```python
from build123d import *

# Parameters (mm, degrees)
HOLE1_D                      = 40
HOLE1_CBORE_D                = 70
HOLE1_CBORE_DEPTH            = 15
SKETCH4_R                    = 68
SKETCH4_R_2                  = 62
CUT_EXTRUDE1_DEPTH           = 3
FILLET1_R                    = 21
FILLET2_R                    = 12
BOSS_EXTRUDE1_START          = -10
BOSS_EXTRUDE1_DEPTH          = 10
CIRPATTERN1_COUNT            = 5
M10_TAPPED_HOLE1_D           = 8.5
M10_TAPPED_HOLE1_DEPTH       = 21.946342369
M10_TAPPED_HOLE1_CSINK_D     = 10.05
M10_TAPPED_HOLE1_CSINK_ANGLE = 90
M10_TAPPED_HOLE1_TIP         = 2.553657631


with BuildPart() as part:
    # Sketch1 → Revolve1 (revolve)
    with BuildSketch(Plane.XY, mode=Mode.PRIVATE) as revolve1_sk:
        Polygon((0, 0), (0, 90), (-85, 90), (-85, 80), (-40, 80), (-40, 6), (-50, 6), (-50, 0), align=None)
    revolve(revolve1_sk.sketch.rotate(Axis((0, 0, 0), (0, 1, 0)), 270), axis=Axis((0, 0, 0), (0, 1, 0)))

    # Hole1 (through all)
    with Locations(Plane(origin=(0, 90, 0), x_dir=(1, 0, 0), z_dir=(0, 1, 0))):
        with Locations((0, 0)):
            CounterBoreHole(HOLE1_D / 2, HOLE1_CBORE_D / 2, HOLE1_CBORE_DEPTH)

    # Sketch4 → Cut-Extrude1 (cut)
    with BuildSketch(Plane(origin=(0, 90, 0), x_dir=(1, 0, 0), z_dir=(0, 1, 0))):
        with Locations(Location((0, 0, 0), (0, 0, 270))):
            Circle(SKETCH4_R)
        with Locations(Location((0, 0, 0), (0, 0, 270))):
            Circle(SKETCH4_R_2, mode=Mode.SUBTRACT)
    extrude(amount=-CUT_EXTRUDE1_DEPTH, mode=Mode.SUBTRACT)

    # Fillet1
    fillet1_edges = [part.edges().sort_by_distance(p)[0] for p in [
        (0, 80, 40),
    ]]
    fillet(fillet1_edges, radius=FILLET1_R)

    # Fillet2
    # the kernel refuses this fillet: 12 mm, written as the material it adds along each edge
    with BuildSketch(Plane(origin=(0, 6, 0), x_dir=(0, 0, -1), z_dir=(1, 0, 0))) as fillet2_piece_1:
        with BuildLine():
            CenterArc((52, 11.832159566), FILLET2_R, 180, 80.405931773)
            Line((50, 0), (49.96, -0.236643191))
            ThreePointArc((49.96, -0.236643191), (45, -0.24), (40, -0.24))
            Line((40, -0.24), (39.76, 0))
            Line((39.76, 0), (39.76, 11.832159566))
            Line((39.76, 11.832159566), (40, 11.832159566))
        make_face()
    revolve(axis=Axis((0, 6, 0), (0, 1, 0)))

    # Sketch5 → Boss-Extrude1 (add)
    with BuildSketch(Plane(origin=(0, 90, 0), x_dir=(1, 0, 0), z_dir=(0, 1, 0)).offset(BOSS_EXTRUDE1_START)):
        with BuildLine():
            ThreePointArc((12.466163113, 84.080882353), (0, 97.5), (-12.466163113, 84.080882353))
            ThreePointArc((-12.466163113, 84.080882353), (0, 85), (12.466163113, 84.080882353))
        make_face()
    boss_extrude1 = extrude(amount=BOSS_EXTRUDE1_DEPTH)

    # CirPattern1: Boss-Extrude1 ×5 about axis
    cirpattern1_axis = Axis((0, 0, 0), (0, 1, 0))
    for i in range(1, CIRPATTERN1_COUNT):
        add(boss_extrude1.rotate(cirpattern1_axis, i * 360 / CIRPATTERN1_COUNT))

    # M10 Tapped Hole1
    with Locations(Plane(origin=(0, 90, 0), x_dir=(1, 0, 0), z_dir=(0, 1, 0))):
        with Locations((49.961746445, -68.766444522), (-49.961746445, -68.766444522), (80.839803885, 26.266444522), (0, 85), (-80.839803885, 26.266444522)):
            CounterSinkHole(M10_TAPPED_HOLE1_D / 2, M10_TAPPED_HOLE1_CSINK_D / 2, depth=M10_TAPPED_HOLE1_DEPTH, counter_sink_angle=M10_TAPPED_HOLE1_CSINK_ANGLE)
            with Locations((0, 0, -(M10_TAPPED_HOLE1_DEPTH + M10_TAPPED_HOLE1_TIP / 2))):  # 118° drill point
                Cone(0, M10_TAPPED_HOLE1_D / 2, M10_TAPPED_HOLE1_TIP, mode=Mode.SUBTRACT)


solid = part.part
```
CAD build for the part. Positions are in the model's coordinates, mm. A direction names the side the tool comes from. Give positions to 0.01 mm unless a question says otherwise; leave off trailing zeros. Loops run counter-clockwise (first coordinate to the right, second up) from the corner with the lowest first, then second, coordinate; pieces in that order, holes last. Notation, with made-up numbers: M -33,-17.75 L -18,-17.75 A28 cw -18,16.25 Z; hole C 9.25,25.25 d5. An arc over 180 degrees is marked long. Use one line per item in the form item = value.
Item 1: Slice it at D-D (y = 69). List the corners of the cut face in (x, z).
Determined:
outline = C 0,0 d85.07; hole C 0,0 d40
Item 2: Which spindle directions (+Z, -Z, +X, -X, +Y, -Y) get a long thin tool onto all of the face, cutting with end or side? Do faces 1 (the face through (67.42, 88.52, -8.85)), 2 (the face through (-15.02, 2.96, -47.69)), 3 (the face through (-42, 90, 54)). Say none if no direction does.
Determined:
face_1 = +Y
face_2 = -Y
face_3 = +Z, -Z, +X, -X, +Y
Item 3: Drill centre lines: probe 1 along X at (y, z) = (84, -85); probe 2 along Z at (x, y) = (0, 56); probe 3 along Y at (x, z) = (-65.5, 7). Where is each one in solid material? Low to high. Write a range as from..to.
Determined:
probe_1 = -12.5..-4.25, 4.25..12.5
probe_2 = -40..-20, 20..40
probe_3 = 80..87
Item 4: Two-plate mould, pull along Z, no slides. Class faces 4 (the face through (27, 90, 27)), 5 (the face through (39.05, 38.13, 8.67)), 6 (the face through (15, 75, 15)), 7 (the face through (-49.5, 84.9, -69.1)): pulls with the +Z half, pulls with the -Z half, needs draft (parallel to the pull), parting line crosses it, or undercut.
Determined:
face_4 = needs draft
face_5 = parting line crosses it
face_6 = undercut
face_7 = pulls with the -Z half
Item 5: Slice it at B-B (x = 0). Count the separate pieces of the cut face and the enclosed holes in it, plus the area to 3 significant figures.
Determined:
separate_pieces = 3
enclosed_holes = 0
area = 4,420 mm2
Item 6: Slice it at C-C (y = 11.5). List the corners of the cut face in (x, z), plus the area to 3 significant figures.
Determined:
outline = C 0,0 d83.61; hole C 0,0 d40
area = 4,230 mm2
Item 7: Flat gauge pins, fed straight in: pin 1 (12 mm diameter, centred on x = -14, y = 19, fed in from -Z); pin 2 (11 mm diameter, centred on x = 0, z = -85, fed in from -Y); pin 3 (7 mm diameter, centred on x = 49.96, z = 68.77, fed in from +Y); pin 4 (8 mm diameter, centred on y = 11.5, z = 2.5, fed in from +X). Where does each tip first touch, or does it go through?
Determined:
pin_1 = -39.21
pin_2 = 80
pin_3 = through
pin_4 = 45.83
